Verification items for the finished model (mm, model axes). Give positions to 0.01 mm unless a question says otherwise; leave off trailing zeros. Order: outer loops, then holes, each group sorted by start corner. A loop starts at its lowest first (then second) coordinate and runs counter-clockwise, first axis right, second up. Notation, with made-up numbers: (17, -14) -> (61, -14) arc R6 cw to (61, -6) -> close; hole circle Ø7 at (-23, 9.25). An arc over 180 degrees is marked (long way). Write each question's results on one line, items separated by ' | '. Start each with the question number.
1. Depth check by flat-ended pin: pin 1 Ø8.5 at (y, z) = (0, 76.2) entering from +X. Enter the tip coordinate at first touch or a pass-through.
2. Cross-section at A-A, the plane y = 0. Enter the section's corners in (x, z) (3 decimals).
3. Cross-section at B-B, the plane z = -127. Enter the section's corners in (x, y) (3 decimals).
4. Material ranges on L1, parallel to Z at x = 5.5, y = 0 (3 decimals); L2, parallel to Z at x = 9.25, y = 1.5; L3, parallel to Y at x = 1.75, z = 76.2 (3 decimals), recorded low to high. Write a range as from..to.
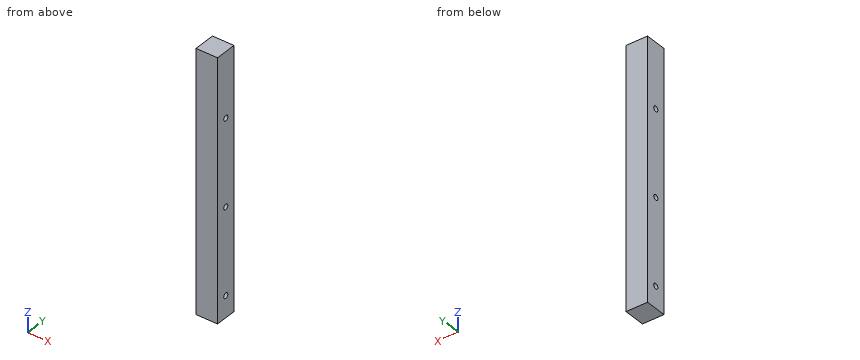
from build123d import *

# Parameters (mm, degrees)
SKETCH7_W           = 25.4
SKETCH7_H           = 25.4
BOSS_EXTRUDE3_DEPTH = 152.4
SKETCH9_R           = 3.175
CUT_EXTRUDE1_DEPTH  = 156.02325632
LPATTERN1_COUNT     = 2
LPATTERN1_PITCH     = 101.6
LPATTERN1_COL_COUNT = 2
LPATTERN1_COL_PITCH = 101.6


with BuildPart() as part:
    # Sketch7 → Boss-Extrude3 (new, symmetric)
    with BuildSketch(Plane.XY):
        Rectangle(SKETCH7_W, SKETCH7_H)
    extrude(amount=BOSS_EXTRUDE3_DEPTH, both=True)

    # Sketch9 → Cut-Extrude1 (cut, through all)
    with BuildSketch(Plane(origin=(12.7, 0, 0), x_dir=(0, -1, 0), z_dir=(-1, 0, 0))):
        with Locations(Location((0, -25.4, 0), (0, 0, 90))):
            Circle(SKETCH9_R)
    cut_extrude1 = extrude(amount=CUT_EXTRUDE1_DEPTH, mode=Mode.SUBTRACT)

    # LPattern1: Cut-Extrude1 ×2
    with Locations(*[(0, 0, -i * LPATTERN1_PITCH) for i in range(1, LPATTERN1_COUNT)]):
        add(cut_extrude1, mode=Mode.SUBTRACT)

    # LPattern1 col: Cut-Extrude1 ×2
    with Locations(*[(0, 0, i * LPATTERN1_COL_PITCH) for i in range(1, LPATTERN1_COL_COUNT)]):
        add(cut_extrude1, mode=Mode.SUBTRACT)


solid = part.part
Results below:
1) pin 1: stops at x = 12.7
2) outline: (-12.7, -152.4) -> (12.7, -152.4) -> (12.7, -130.175) -> (-12.7, -130.175) -> close; (-12.7, -123.825) -> (12.7, -123.825) -> (12.7, -28.575) -> (-12.7, -28.575) -> close; (-12.7, -22.225) -> (12.7, -22.225) -> (12.7, 73.025) -> (-12.7, 73.025) -> close; (-12.7, 79.375) -> (12.7, 79.375) -> (12.7, 152.4) -> (-12.7, 152.4) -> close
3) outline: (-12.7, -12.7) -> (12.7, -12.7) -> (12.7, -3.175) -> (-12.7, -3.175) -> close; (-12.7, 3.175) -> (12.7, 3.175) -> (12.7, 12.7) -> (-12.7, 12.7) -> close
4) L1: z = -152.4..-130.175, -123.825..-28.575, -22.225..73.025, 79.375..152.4 | L2: z = -152.4..-129.8, -124.2..-28.2, -22.6..73.4, 79..152.4 | L3: y = -12.7..-3.175, 3.175..12.7
